Verification items for this drawing (mm, ordinates from the low corner). Give positions to 0.01 mm unless a question says otherwise; leave off trailing zeros. Order: outer loops, then holes, each group sorted by start corner. A loop starts at its lowest first (then second) coordinate and runs counter-clockwise, first axis right, second up. Notation, with made-up numbers: (75.5, 71) - (93.5, 71) arc R15 cw to (93.5, 100) - close; hole circle Ø11 at (65.5, -0.75). An arc over 180 degrees is marked (long way). Put each result on its own line as item: value. Start each with the question number.
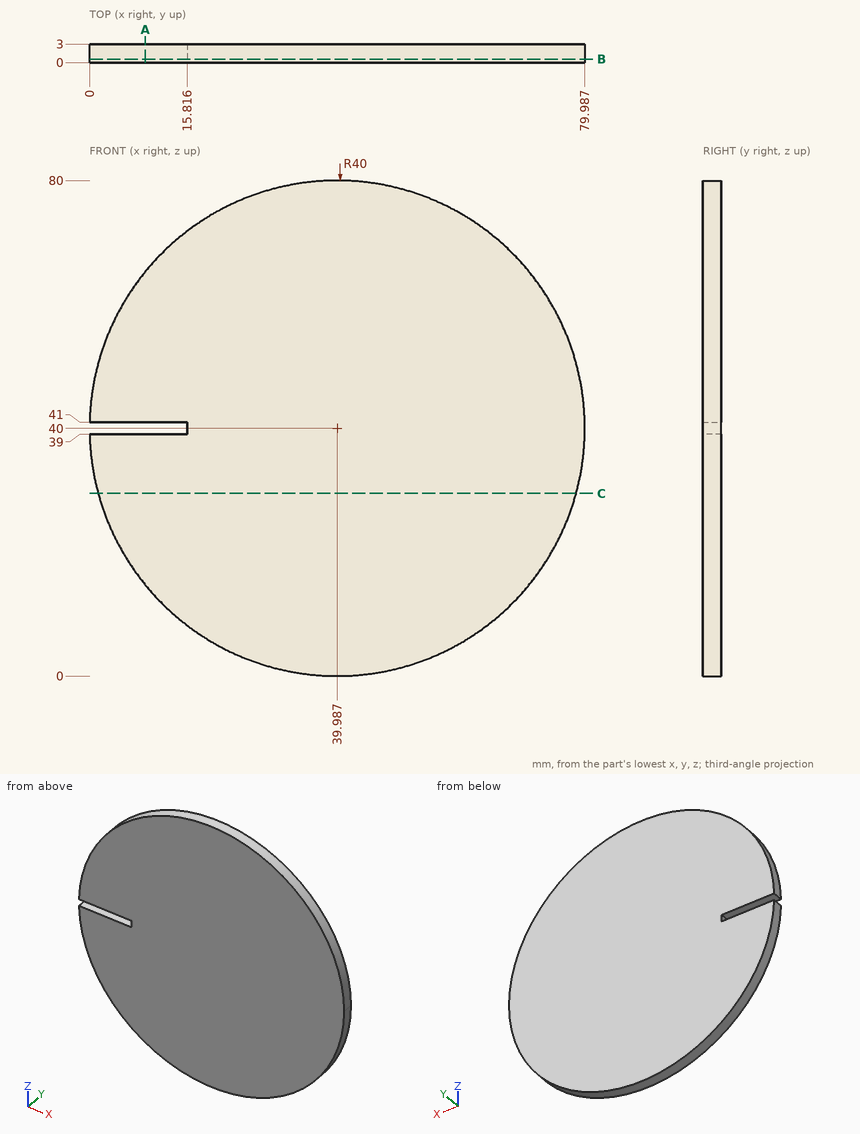
Item 1: Cross-section at A-A (x = 9). Enter the section's corners in (y, z).
Item 2: Thickness scan on line 1 along X through (y, z) = (1.85, 40); line 2 along Z through (x, y) = (7, 1.7) (1 decimal); line 3 along X through (y, z) = (2.7, 65) (1 decimal). Record the ranges inside material, lowest first.
Item 3: Gauge pin test, flat ends, axial feed: pin 1 Ø1.5 at (y, z) = (2, 26.5) entering from -X; pin 2 Ø0.9 at (x, y) = (8.5, 2) entering from -Z; pin 3 Ø1.5 at (y, z) = (1.5, 21.5) entering from -X. Record the tip position at first contact, or that the pin passes through.
Item 4: Cross-section at B-B (y = 0.55). Enter the section's corners in (x, z).
Item 5: Cross-section at C-C (z = 29.5). Enter the section's corners in (x, y) (1 decimal).
Recorded:
1. outline: (0, 14.71) - (3, 14.71) - (3, 39) - (0, 39) - close; (0, 41) - (3, 41) - (3, 65.29) - (0, 65.29) - close
2. line 1: x = 15.82 to 79.99
2. line 2: z = 17.4 to 39, 41 to 62.6
2. line 3: x = 8.8 to 71.2
3. pin 1: stops at x = 2.07
3. pin 2: stops at z = 14.77
3. pin 3: stops at x = 4.14
4. outline: (0, 39) arc R40 ccw (long way) to (0, 41) - (15.82, 41) - (15.82, 39) - close
5. outline: (1.4, 0) - (78.6, 0) - (78.6, 3) - (1.4, 3) - close
